For this review, take the finished solid that the model builds, in its own axes (mm). Face numbers are marked on the shaded views. Round coordinates to 2 decimals unless told otherwise and drop trailing zeros. Order: outer loops, then holes, each group sorted by start corner. A loop starts at its lowest first (then second) coordinate and runs counter-clockwise, first axis right, second up. Notation, with made-up numbers: (-15, 59.5) - (33, 59.5) arc R17 ccw to (33, 80.5) - close; hole circle Ø4 at (30, -38.75). An arc over 180 degrees is marked (long way). One line per item, written item: value.
```python
from build123d import *

# Parameters (mm, degrees)
F1_DEPTH = 1.5
F2_W     = 10
F2_H     = 3.2
F3_DEPTH = 3.001


with BuildPart() as f1:
    # F0 (on Front) → F1 (new body, symmetric)
    with BuildSketch(Plane.XZ):
        with BuildLine():
            Line((0, -35), (0, 0))
            Line((0, 0), (-50, 0))
            Line((-50, 0), (-90, -40))
            Line((-90, -40), (-90, -170))
            Line((-90, -170), (-50, -210))
            Line((-50, -210), (-21.715729, -181.715729))
            Line((-21.715729, -181.715729), (-50, -153.431458))
            Line((-50, -153.431458), (-50, -85))
            ThreePointArc((-50, -85), (-35.355339, -49.644661), (0, -35))
        make_face()
    extrude(amount=F1_DEPTH, both=True)

    # F2 (on face) → F3 (cut, through all)
    with BuildSketch(Plane.XZ.offset(1.5)):
        with BuildLine():
            Line((0, 0), (-20, 0))
            Line((-20, 0), (-20, -10))
            Line((-20, -10), (-30, -10))
            Line((-30, -10), (-30, -13.2))
            Line((-30, -13.2), (-20, -13.2))
            Line((-20, -13.2), (-20, -39.174243))
            ThreePointArc((-20, -39.174243), (-10.215482, -36.054684), (0, -35))
            Line((0, -35), (0, 0))
        make_face()
        with Locations((-55, -148.4)):
            Rectangle(F2_W, F2_H)
    extrude(amount=-F3_DEPTH, mode=Mode.SUBTRACT)


solid = f1.part
```
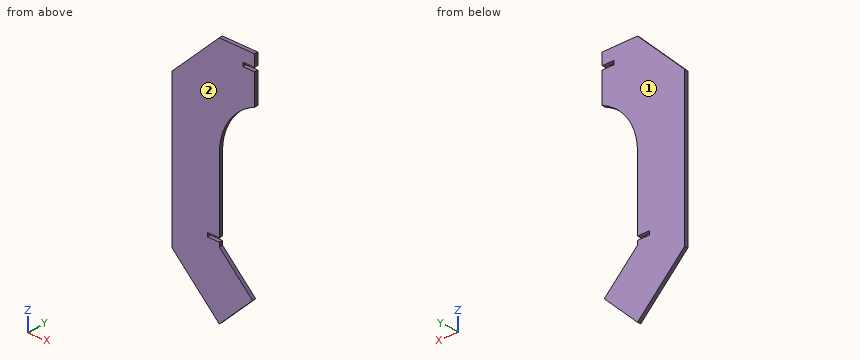
Item 1: Take a section at A-A (x = -54.5). Write out the cut boundary in (y, z).
Returned:
outline: (-1.5, -205.5) - (1.5, -205.5) - (1.5, -150) - (-1.5, -150) - close; (-1.5, -146.8) - (1.5, -146.8) - (1.5, -4.5) - (-1.5, -4.5) - close
Item 2: Wall thickness on line 1 (Z direction, x = -26.5, y = -1.1); line 2 (X direction, y = 0.3, z = -105.5); line 3 (Z direction, x = -41, y = -0.35): over which ranges is each line inside the solid? List them lowest first.
Returned:
line 1: -186.5 to -176.93, -42.6 to -13.2, -10 to 0
line 2: -90 to -50
line 3: -201 to -162.43, -56.38 to 0
Item 3: Take a section at B-B (y = -0.5). Write out the cut boundary in (x, z), plus the area to 3 significant figures.
Returned:
outline: (-90, -170) - (-50, -210) - (-21.72, -181.72) - (-50, -153.43) - (-50, -150) - (-60, -150) - (-60, -146.8) - (-50, -146.8) - (-50, -85) arc R50 cw to (-20, -39.17) - (-20, -13.2) - (-30, -13.2) - (-30, -10) - (-20, -10) - (-20, 0) - (-50, 0) - (-90, -40) - close
area: 9,100 mm^2
Item 4: Take a section at D-D (x = -67). Write out the cut boundary in (y, z), plus the area to 3 significant figures.
Returned:
outline: (-1.5, -193) - (1.5, -193) - (1.5, -17) - (-1.5, -17) - close
area: 528 mm^2
Item 5: The part is to be moulded in two halves that separate along Y. For the marked faces 1 and 2, say which applies: +Y half, -Y half, draft (parallel to the pull), parting line (faces both ways), or undercut.
Returned:
face 1: +Y half
face 2: -Y half
Item 6: For P1, Ø1.5, axis at x = -23.5, y = 0.5, coming from the -Z side; P2, Ø1.5, axis at y = 0.5, z = -12, coming from the +X side; P3, Ø1.5, axis at x = -57, y = 0.5, coming from the +Z side, all flat-tipped, find the tip position at first contact; note any pin that passes through.
Returned:
P1: z = -184.25
P2: x = -30
P3: z = -6.25
Item 7: Take a section at C-C (z = -21.5). Write out the cut boundary in (x, y).
Returned:
outline: (-71.5, -1.5) - (-20, -1.5) - (-20, 1.5) - (-71.5, 1.5) - close
